Source: CAD feature listing. Evaluate the final solid. Frame: model axes, mm. Face numbers are marked on the shaded views. A direction names the side the tool comes from. Round coordinates to 2 decimals unless told otherwise and drop trailing zeros. Order: outer loops, then holes, each group sorted by start corner. A loop starts at its lowest first (then second) coordinate and runs counter-clockwise, first axis right, second up. Notation, with made-up numbers: (78, -31.75) -> (93, -31.75) arc R26 cw to (93, -5.75) -> close; hole circle Ø5 at (35, 35.25). An arc over 180 degrees is marked (long way). One line per item, written item: value. Start each with the question number.
1) Section C-C (y = 12). Return the cut outline in (x, z), and give its area (3 significant figures).
2) Section A-A (x = 13). Return the cut outline in (y, z).
3) Section D-D (z = 11). Return the cut outline in (x, y).
4) Reachability of the marked faces 1, 2 and 3 from +Z, -Z, +X, -X, +Y, -Y: full face, straight path, thin tool, end or side. Return the list, or none.
5) Pin query (flat end, axial travel): P1, Ø4, axis at x = 0.5, z = -9.5, coming from the -Y side; P2, Ø4, axis at x = 13, z = 24.75, coming from the +Y side; P3, Ø1, axis at y = 25.5, z = 1.5, coming from the +X side. Return the tip coordinate at first contact, or that it passes through.
6) Ray query, L1, parallel to Z at x = 13, y = 2.4; L2, parallel to Y at x = 0.75, z = -22; L3, parallel to Y at x = -3, z = -8. Return the intervals inside material, ascending.
7) Section B-B (y = 34.1). Return the cut outline in (x, z), and give its area (3 significant figures).
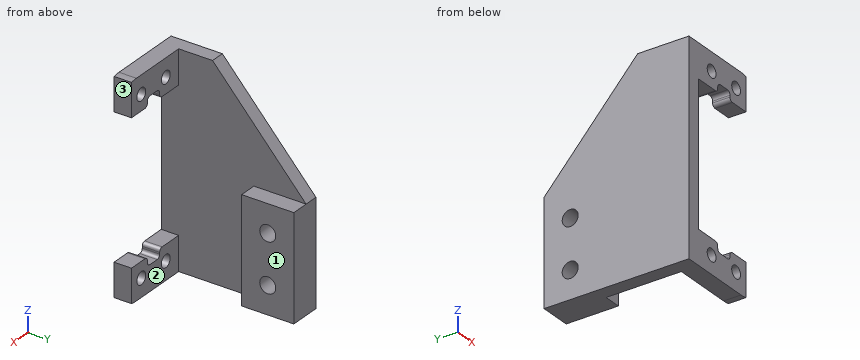
```python
from build123d import *

# Parameters (mm, degrees)
SKETCH1_W           = 50
SKETCH1_H           = 60
BOSS_EXTRUDE1_DEPTH = 5
SKETCH2_W           = 20.5
SKETCH2_H           = 40.5
CUT_EXTRUDE1_DEPTH  = 5
SKETCH3_R           = 1.8
CUT_EXTRUDE2_DEPTH  = 5
SKETCH4_R           = 2.5
CUT_EXTRUDE3_DEPTH  = 5
FILLET1_R           = 10
SKETCH5_W           = 5
SKETCH5_H           = 5
CUT_EXTRUDE4_DEPTH  = 10
FILLET2_R           = 1
SKETCH6_W           = 17.943789306
SKETCH6_H           = 60
CUT_EXTRUDE5_DEPTH  = 10
SKETCH7_W           = 4
SKETCH7_H           = 60
BOSS_EXTRUDE2_DEPTH = 36.6
SKETCH8_W           = 21.864927769
SKETCH8_H           = 69.948880873
CUT_EXTRUDE6_DEPTH  = 24
SKETCH9_W           = 30
SKETCH9_H           = 15
BOSS_EXTRUDE3_DEPTH = 5
CUT_EXTRUDE7_DEPTH  = 5
SKETCH11_R          = 2.3
CUT_EXTRUDE8_DEPTH  = 13


with BuildPart() as part:
    # Sketch1 → Boss-Extrude1 (new body)
    with BuildSketch(Plane(origin=(0, 0, 0), x_dir=(1, 0, 0), z_dir=(0, 1, 0))):
        Rectangle(SKETCH1_W, SKETCH1_H)
    extrude(amount=BOSS_EXTRUDE1_DEPTH)

    # Sketch2 → Cut-Extrude1 (cut)
    with BuildSketch(Plane(origin=(0, 5, 0), x_dir=(1, 0, 0), z_dir=(0, 1, 0))):
        with Locations((8, 0)):
            Rectangle(SKETCH2_W, SKETCH2_H)
    extrude(amount=-CUT_EXTRUDE1_DEPTH, mode=Mode.SUBTRACT)

    # Sketch3 → Cut-Extrude2 (cut)
    with BuildSketch(Plane(origin=(0, 5, 0), x_dir=(1, 0, 0), z_dir=(0, 1, 0))):
        with Locations((3, 24.75)):
            Circle(SKETCH3_R)
        with Locations((13, 24.75)):
            Circle(SKETCH3_R)
        with Locations((13, -24.75)):
            Circle(SKETCH3_R)
        with Locations((3, -24.75)):
            Circle(SKETCH3_R)
    extrude(amount=-CUT_EXTRUDE2_DEPTH, mode=Mode.SUBTRACT)

    # Sketch4 → Cut-Extrude3 (cut)
    with BuildSketch(Plane(origin=(0, 5, 0), x_dir=(1, 0, 0), z_dir=(0, 1, 0))):
        with Locations((-17.5, 20)):
            Circle(SKETCH4_R)
        with Locations((-17.5, -20)):
            Circle(SKETCH4_R)
    extrude(amount=-CUT_EXTRUDE3_DEPTH, mode=Mode.SUBTRACT)

    # Fillet1
    fillet1_edges = [part.edges().sort_by_distance(p)[0] for p in [
        (-25, 2.5, -30),
        (25, 2.5, -30),
        (25, 2.5, 30),
        (-25, 2.5, 30),
    ]]
    fillet(fillet1_edges, radius=FILLET1_R)

    # Sketch5 → Cut-Extrude4 (cut)
    with BuildSketch(Plane(origin=(0, 5, 0), x_dir=(1, 0, 0), z_dir=(0, 1, 0))):
        with Locations((8, 20.25)):
            Rectangle(SKETCH5_W, SKETCH5_H)
    cut_extrude4 = extrude(amount=-CUT_EXTRUDE4_DEPTH, mode=Mode.SUBTRACT)

    # Mirror1: Cut-Extrude4 across plane
    add(cut_extrude4.mirror(Plane.XY), mode=Mode.SUBTRACT)

    # Fillet2
    fillet2_edges = [part.edges().sort_by_distance(p)[0] for p in [
        (10.5, 2.5, 20.25),
        (5.5, 2.5, 20.25),
        (10.5, 2.5, 22.75),
        (5.5, 2.5, 22.75),
        (10.5, 2.5, -20.25),
        (5.5, 2.5, -20.25),
        (5.5, 2.5, -22.75),
        (10.5, 2.5, -22.75),
    ]]
    fillet(fillet2_edges, radius=FILLET2_R)

    # Sketch6 → Cut-Extrude5 (cut)
    with BuildSketch(Plane(origin=(0, 5, 0), x_dir=(1, 0, 0), z_dir=(0, 1, 0))):
        with Locations((25.971894653, 0)):
            Rectangle(SKETCH6_W, SKETCH6_H)
    extrude(amount=-CUT_EXTRUDE5_DEPTH, mode=Mode.SUBTRACT)

    # Sketch7 → Boss-Extrude2 (add)
    with BuildSketch(Plane(origin=(0, 5, 0), x_dir=(1, 0, 0), z_dir=(0, 1, 0))):
        with Locations((-4.25, 0)):
            Rectangle(SKETCH7_W, SKETCH7_H)
    extrude(amount=BOSS_EXTRUDE2_DEPTH)

    # Sketch8 → Cut-Extrude6 (cut)
    with BuildSketch(Plane(origin=(0, 5, 0), x_dir=(1, 0, 0), z_dir=(0, 1, 0))):
        with Locations((-17.182463885, 4.974440436)):
            Rectangle(SKETCH8_W, SKETCH8_H)
    extrude(amount=-CUT_EXTRUDE6_DEPTH, mode=Mode.SUBTRACT)

    # Sketch9 → Boss-Extrude3 (add)
    with BuildSketch(Plane(origin=(-2.25, 0, 0), x_dir=(0, 0, -1), z_dir=(1, 0, 0))):
        with Locations((15, 34.1)):
            Rectangle(SKETCH9_W, SKETCH9_H)
    extrude(amount=BOSS_EXTRUDE3_DEPTH)

    # Sketch10 → Cut-Extrude7 (cut)
    with BuildSketch(Plane(origin=(-2.25, 0, 0), x_dir=(0, 0, -1), z_dir=(1, 0, 0))):
        Polygon((0, 41.6), (-30, 14.728132264), (-30, 41.6), align=None)
    extrude(amount=-CUT_EXTRUDE7_DEPTH, mode=Mode.SUBTRACT)

    # Sketch11 → Cut-Extrude8 (cut)
    with BuildSketch(Plane(origin=(2.75, 0, 0), x_dir=(0, 0, -1), z_dir=(1, 0, 0))):
        with Locations((8, 34.1)):
            Circle(SKETCH11_R)
        with Locations((22, 34.1)):
            Circle(SKETCH11_R)
    extrude(amount=-CUT_EXTRUDE8_DEPTH, mode=Mode.SUBTRACT)


solid = part.part
```
Findings:
1. outline: (-6.25, -30) -> (-2.25, -30) -> (-2.25, 30) -> (-6.25, 30) -> close
1. area: 240 mm2
2. outline: (0, -30) -> (5, -30) -> (5, -26.55) -> (0, -26.55) -> close; (0, -22.95) -> (5, -22.95) -> (5, -20.25) -> (0, -20.25) -> close; (0, 20.25) -> (5, 20.25) -> (5, 22.95) -> (0, 22.95) -> close; (0, 26.55) -> (5, 26.55) -> (5, 30) -> (0, 30) -> close
3. outline: (-6.25, 0) -> (-2.25, 0) -> (-2.25, 31.75) -> (-6.25, 31.75) -> close
4. face 1: +Z, -Z, +X, +Y
4. face 2: +Z, -Z, +X
4. face 3: +Z, -Z, +X, +Y, -Y
5. P1: y = 26.6
5. P2: y = 5
5. P3: x = -2.25
6. L1: -30 to -26.55, -22.95 to -20.25, 20.25 to 22.95, 26.55 to 30
6. L2: 0 to 5, 26.6 to 31.8, 36.4 to 41.6
6. L3: 0 to 31.8, 36.4 to 41.6
7. outline: (-6.25, -30) -> (2.75, -30) -> (2.75, -24.3) -> (-6.25, -24.3) -> close; (-6.25, -19.7) -> (2.75, -19.7) -> (2.75, -10.3) -> (-6.25, -10.3) -> close; (-6.25, -5.7) -> (2.75, -5.7) -> (2.75, 0) -> (-2.25, 0) -> (-2.25, 8.37) -> (-6.25, 8.37) -> close
7. area: 221 mm2
